Verification items for the finished model (mm, model axes). A direction names the side the tool comes from. Give positions to 0.01 mm unless a question says otherwise; leave off trailing zeros. Order: outer loops, then holes, each group sorted by start corner. A loop starts at its lowest first (then second) coordinate and runs counter-clockwise, first axis right, second up. Notation, with made-up numbers: (27, 57.25) - (84, 57.25) arc R21 cw to (84, 84.25) - close; hole circle Ø3 at (36.25, 6). An arc over 180 degrees is marked (long way). Answer as a JSON object with one key per item and string values.
```python
from build123d import *

# Parameters (mm, degrees)
BOSS_EXTRUDE1_DEPTH = 1.3
FILLET1_R           = 2
BOSS_EXTRUDE2_DEPTH = 0.5


with BuildPart() as part:
    # Sketch1 → Boss-Extrude1 (new body)
    with BuildSketch(Plane(origin=(0, 0, 0), x_dir=(1, 0, 0), z_dir=(0, 1, 0))):
        with BuildLine():
            ThreePointArc((-34.363462402, 3.807782606), (-31.263462402, 10.335627538), (-28.163462402, 3.807782606))
            Line((-28.163462402, 3.807782606), (-28.163462402, -1.578916037))
            ThreePointArc((-28.163462402, -1.578916037), (-27.18017283, -1.119353768), (-26.263462402, -0.538236004))
            Line((-26.263462402, -0.538236004), (-26.263462402, 2.182315607))
            ThreePointArc((-26.263462402, 2.182315607), (-24.763462402, 6.335627538), (-26.263462402, 10.488939469))
            Line((-26.263462402, 10.488939469), (-26.263462402, 13.20949108))
            ThreePointArc((-26.263462402, 13.20949108), (-31.263462402, 14.835627538), (-36.263462402, 13.20949108))
            Line((-36.263462402, 13.20949108), (-36.263462402, 10.488939469))
            ThreePointArc((-36.263462402, 10.488939469), (-37.763462402, 6.335627538), (-36.263462402, 2.182315607))
            Line((-36.263462402, 2.182315607), (-36.263462402, -0.538236004))
            ThreePointArc((-36.263462402, -0.538236004), (-35.346751974, -1.119353768), (-34.363462402, -1.578916037))
            Line((-34.363462402, -1.578916037), (-34.363462402, 3.807782606))
        make_face()
        with BuildLine():
            Line((-28.163462402, 13.16497597), (-28.163462402, 12.048770281))
            ThreePointArc((-28.163462402, 12.048770281), (-31.263462402, 12.835627538), (-34.363462402, 12.048770281))
            Line((-34.363462402, 12.048770281), (-34.363462402, 13.16497597))
            ThreePointArc((-34.363462402, 13.16497597), (-31.263462402, 13.835627538), (-28.163462402, 13.16497597))
        make_face(mode=Mode.SUBTRACT)
    extrude(amount=BOSS_EXTRUDE1_DEPTH)

    # Fillet1
    # the kernel refuses this fillet: 2 mm, written as the material it takes off along each edge
    with BuildSketch(Plane(origin=(-34.363462402, -7.59544617, 1.578916037), x_dir=(-0.877056624193214, 0, -0.4803870085241726), z_dir=(0, 1, 0))) as fillet1_piece_1:
        with BuildLine():
            CenterArc((3.213614714, -1.703880534), FILLET1_R, 121.576665182, 87.134016017)
            Line((1.459501466, -2.664654551), (1.424419201, -2.683870031))
            Line((1.424419201, -2.683870031), (-0.035082265, -0.01921548))
            Line((-0.035082265, -0.01921548), (-0.005097263, 0.039673895))
            ThreePointArc((-0.005097263, 0.039673895), (1.083168377, 0.109297404), (2.145391194, 0.034077611))
            Line((2.145391194, 0.034077611), (2.166336754, 0))
        make_face()
    extrude(amount=16.49089234, mode=Mode.SUBTRACT)
    with BuildSketch(Plane(origin=(-28.163462402, -7.59544617, 1.578916037), x_dir=(0, 0, -1), z_dir=(0, 1, 0))) as fillet1_piece_2:
        with BuildLine():
            CenterArc((3.038178468, -2), FILLET1_R, 90, 87.134016017)
            Line((1.040680033, -1.9), (1.000730064, -1.898))
            ThreePointArc((1.000730064, -1.898), (0.424480004, -1.002505053), (-0.037244911, -0.014588235))
            Line((-0.037244911, -0.014588235), (0, 0.04))
            Line((0, 0.04), (3.038178468, 0.04))
            Line((3.038178468, 0.04), (3.038178468, 0))
        make_face()
    extrude(amount=16.49089234, mode=Mode.SUBTRACT)

    # Sketch2 → Boss-Extrude2 (add)
    with BuildSketch(Plane(origin=(0, 1.3, 0), x_dir=(1, 0, 0), z_dir=(0, 1, 0))):
        with BuildLine():
            Line((-26.263462402, 12.70949108), (-26.263462402, 13.20949108))
            ThreePointArc((-26.263462402, 13.20949108), (-31.263462402, 14.835627538), (-36.263462402, 13.20949108))
            Line((-36.263462402, 13.20949108), (-36.263462402, 12.70949108))
            ThreePointArc((-36.263462402, 12.70949108), (-31.263462402, 14.464493082), (-26.263462402, 12.70949108))
        make_face()
    extrude(amount=BOSS_EXTRUDE2_DEPTH)


solid = part.part
```
(1) Section check C-C (y = 0.4). Record the cut outline in (x, z), then the cut area to 3 significant figures.
Computed values:
{"outline": "(-36.26, -13.21) arc R8.5 ccw to (-26.26, -13.21) - (-26.26, -10.49) arc R6.5 ccw to (-26.26, -2.18) - (-26.26, 0.54) arc R2 ccw to (-28.16, -1.46) - (-28.16, -3.81) arc R4 cw (long way) to (-34.36, -3.81) - (-34.36, -1.46) arc R2 ccw to (-36.26, 0.54) - (-36.26, -2.18) arc R6.5 ccw to (-36.26, -10.49) - close; hole (-34.36, -13.16) arc R7.5 ccw to (-28.16, -13.16) - (-28.16, -12.05) arc R6.5 cw to (-34.36, -12.05) - close", "area": "86.6 mm²"}
(2) Section check A-A (x = -34). Record the cut outline in (y, z).
Computed values:
{"outline": "(0, -14.38) - (1.8, -14.38) - (1.8, -13.98) - (1.3, -13.98) - (1.3, -13.32) - (0, -13.32) - close; (0, -12.23) - (1.3, -12.23) - (1.3, -9.25) - (0, -9.25) - close"}
(3) Section check D-D (x = -28.75). Record the cut outline in (y, z).
Computed values:
{"outline": "(0, -14.46) - (1.8, -14.46) - (1.8, -14.06) - (1.3, -14.06) - (1.3, -13.4) - (0, -13.4) - close; (0, -12.33) - (1.3, -12.33) - (1.3, -9.45) - (0, -9.45) - close"}
(4) Section check B-B (z = -8.25). Record the cut outline in (x, y), then the cut area to 3 significant figures.
Computed values:
{"outline": "(-37.48, 0) - (-34.78, 0) - (-34.78, 1.3) - (-37.48, 1.3) - close; (-27.75, 0) - (-25.05, 0) - (-25.05, 1.3) - (-27.75, 1.3) - close", "area": "7.02 mm²"}
(5) Access from +Z, -Z, +X, -X, +Y, -Y to the whole of each face (thin tool, end or side, straight path). Record for faces 4 (the cylindrical face through (-31.339, 1.546, -14.464)), 5 (the flat face through (-28.163, 1, -13)), 6 (the flat face through (-28.163, 1, -3)).
Computed values:
{"face 4": "+Z, +Y", "face 5": "+Y, -Y", "face 6": "+Z, +Y, -Y"}
(6) Gauge pin test, flat ends, axial feed: pin 1 Ø0.9 at (y, z) = (0.5, -12.5) entering from -X; pin 2 Ø6.5 at (x, z) = (-28, -6.5) entering from +Y; pin 3 Ø1 at (x, y) = (-35.5, 1.5) entering from -Z. Record the tip position at first contact, or that the pin passes through.
Computed values:
{"pin 1": "stops at x = -36.26", "pin 2": "stops at y = 1.3", "pin 3": "stops at z = -13.97"}
(7) Material ranges on line 1 along Z through (x, y) = (-31.25, 0.1); line 2 along Y through (x, z) = (-35.25, -2.25); line 3 along X through (y, z) = (1.2, -12), recorded low to high. Write a range as [from, to].
Computed values:
{"line 1": "z = [-14.84, -13.84], [-12.84, -10.34]", "line 2": "y = [0, 1.3]", "line 3": "x = [-36.26, -26.26]"}
(8) Release check for a two-part mould opening along X. For faces 1 (the cylindrical face through (-27.63, 0.64, -0.1)), 2 (the cylindrical face through (-31.189, 0.887, -14.835)), 3 (the flat face through (-36.263, 1, -1)) record: pulls with the +X half, pulls with the -X half, needs draft (parallel to the pull), parting line crosses it, or undercut.
Computed values:
{"face 1": "undercut", "face 2": "parting line crosses it", "face 3": "pulls with the -X half"}
